Geometry check sheet. Reference: the model listing, model coordinates, mm. A direction names the side the tool comes from. Round coordinates to 2 decimals unless told otherwise and drop trailing zeros. Order: outer loops, then holes, each group sorted by start corner. A loop starts at its lowest first (then second) coordinate and runs counter-clockwise, first axis right, second up. Notation, with made-up numbers: (-10, -0.5) - (1, -0.5) arc R17 ccw to (1, 5.5) - close; hole circle Ø5 at (7, 20). An arc over 180 degrees is marked (long way). One line per question, with ' | ' between items. Start each with the question number.
Q1. Sectioned sample at C-C, the plane z = 101. Enter the section's corners in (x, y).
Q2. Sectioned sample at D-D, the plane z = 9. Enter the section's corners in (x, y), then the cut area to 3 significant figures.
Q3. Gauge pin test, flat ends, axial feed: P1, Ø3, axis at x = 4.5, z = 2, coming from the -Y side; P2, Ø1, axis at y = 9.5, z = 49.5, coming from the -X side; P3, Ø3, axis at x = 2, z = 27, coming from the -Y side; P4, Ø1.9, axis at x = 3.5, z = -5, coming from the +Y side. Record the tip position at first contact, or that the pin passes through.
Q4. Material ranges on line 1 along Z through (x, y) = (1, 13.5); line 2 along Y through (x, z) = (3.25, -23.5); line 3 along Y through (x, z) = (1.25, -7), recorded low to high.
Q5. Sectioned sample at A-A, the plane y = 8.5. Enter the section's corners in (x, z).
Q6. Sectioned sample at B-B, the plane x = 3.5. Enter the section's corners in (y, z).
Q7. Tool access check on faces 1 (the face through (3, 55, -110)), 2 (the face through (3, -3, -88.9)), 3 (the face through (3, 61.35, -196)), 4 (the face through (3, -3, 88.9)). Record the directions out of +Z, -Z, +X, -X, +Y, -Y that give a thin tool (end or side, any length) a straight path to the whole face; none if there is none.
Q8. Mould release check, pull along Z, two halves, no side actions. Record for faces 5 (the face through (3, 58, 38.1)), 6 (the face through (3, 61.35, -64)), 7 (the face through (3, 27, 132.7)), 8 (the face through (3, 58, -132.7)): +Z half, -Z half, draft (parallel to the pull), parting line (faces both ways), or undercut.
```python
from build123d import *

# Parameters (mm, degrees)
BOSS_EXTRUDE1_DEPTH = 6.35
SKETCH4_W           = 6.35
SKETCH4_H           = 237.700000096
SKETCH4_H_2         = 112.7
BOSS_EXTRUDE2_DEPTH = 6.35
SKETCH5_W           = 6.35
SKETCH5_H           = 390.400000096
BOSS_EXTRUDE3_DEPTH = 6.35
SKETCH6_W           = 76.2
SKETCH6_H           = 6.35
SKETCH6_W_2         = 43.8
CUT_EXTRUDE1_DEPTH  = 265.978178443


with BuildPart() as part:
    # Sketch3 → Boss-Extrude1 (new body)
    with BuildSketch(Plane(origin=(0, 0, 0), x_dir=(0, 0, -1), z_dir=(1, 0, 0))):
        Polygon((-132.7, 55.000000012), (-132.7, 0), (-20, 0), (-20, 35), (20, 35), (20, 0), (257.700000096, 0), (257.700000096, 55.000000012), align=None)
    extrude(amount=BOSS_EXTRUDE1_DEPTH)

    # Sketch4 → Boss-Extrude2 (add)
    with BuildSketch(Plane.XZ):
        with Locations((3.175, -138.850000048)):
            Rectangle(SKETCH4_W, SKETCH4_H)
        with Locations((3.175, 76.35)):
            Rectangle(SKETCH4_W, SKETCH4_H_2)
    extrude(amount=BOSS_EXTRUDE2_DEPTH)

    # Sketch5 → Boss-Extrude3 (add)
    with BuildSketch(Plane(origin=(0, 55.000000012, 0), x_dir=(1, 0, 0), z_dir=(0, 1, 0))):
        with Locations((3.175, 62.500000048)):
            Rectangle(SKETCH5_W, SKETCH5_H)
    extrude(amount=BOSS_EXTRUDE3_DEPTH)

    # Sketch6 → Cut-Extrude1 (cut, through all)
    with BuildSketch(Plane(origin=(6.35, 0, 0), x_dir=(0, 0, -1), z_dir=(1, 0, 0))):
        Polygon((-132.7, 55.000000012), (-126.35, 55.000000012), (-88.9, 55.000000012), (-88.9, 61.350000012), (-132.7, 61.350000012), align=None)
        Polygon((-88.9, 0), (-126.35, 0), (-132.7, 0), (-132.7, -6.35), (-88.9, -6.35), align=None)
        with Locations((0, 58.175000012)):
            Rectangle(SKETCH6_W, SKETCH6_H)
        Polygon((26.35, 0), (20, 0), (20, -6.35), (38.1, -6.35), (38.1, 0), align=None)
        Polygon((-26.35, 0), (-38.1, 0), (-38.1, -6.35), (-20, -6.35), (-20, 0), align=None)
        with Locations((110.8, 58.175000012)):
            Rectangle(SKETCH6_W_2, SKETCH6_H)
        with Locations((110.8, -3.175)):
            Rectangle(SKETCH6_W_2, SKETCH6_H)
    extrude(amount=-CUT_EXTRUDE1_DEPTH, mode=Mode.SUBTRACT)


solid = part.part
```
Determined:
1) outline: (0, 0) - (6.35, 0) - (6.35, 55) - (0, 55) - close
2) outline: (0, 35) - (6.35, 35) - (6.35, 55) - (0, 55) - close | area: 127 mm2
3) P1: stops at y = 35 | P2: stops at x = 0 | P3: stops at y = 0 | P4: stops at y = 55
4) line 1: z = -257.7 to -20, 20 to 132.7 | line 2: y = 0 to 55 | line 3: y = 35 to 55
5) outline: (0, -257.7) - (6.35, -257.7) - (6.35, -20) - (0, -20) - close; (0, 20) - (6.35, 20) - (6.35, 132.7) - (0, 132.7) - close
6) outline: (-6.35, -257.7) - (61.35, -257.7) - (61.35, -132.7) - (55, -132.7) - (55, -88.9) - (61.35, -88.9) - (61.35, -38.1) - (55, -38.1) - (55, 38.1) - (61.35, 38.1) - (61.35, 88.9) - (55, 88.9) - (55, 132.7) - (0, 132.7) - (0, 88.9) - (-6.35, 88.9) - (-6.35, 38.1) - (0, 38.1) - (0, 20) - (35, 20) - (35, -20) - (0, -20) - (0, -38.1) - (-6.35, -38.1) - (-6.35, -88.9) - (0, -88.9) - (0, -132.7) - (-6.35, -132.7) - close
7) face 1: +X, -X, +Y | face 2: +X, -X, -Y | face 3: +Z, -Z, +X, -X, +Y | face 4: +Z, +X, -X, -Y
8) face 5: undercut | face 6: draft | face 7: +Z half | face 8: undercut
